Could you check a few things on this model? Use its own coordinates, in mm. Face numbers are marked on the shaded views. A direction names the side the tool comes from. Give positions to 0.01 mm unless a question says otherwise; leave off trailing zeros. Loops run counter-clockwise (first coordinate to the right, second up) from the corner with the lowest first, then second, coordinate; pieces in that order, holes last. Notation, with made-up numbers: (-20, 57) - (-13, 57) arc R21 ccw to (-13, 90) - close; hole circle Ø3 at (47.25, 34.5). An arc over 180 degrees is marked (long way). One line per item, written item: value. Start each with the question number.
Q1. I want a section at D-D (y = 30.5). Please give me the cut outline in (x, z), then the cut area to 3 significant figures.
Q2. I want a section at A-A (x = -22). Please give me the cut outline in (y, z), then the cut area to 3 significant figures.
Q3. If I drill on line 1 (Y direction, x = -31.25, z = 0.7); line 2 (Y direction, x = -39, z = 1.05); line 3 (Z direction, x = -53.5, y = 52.5), over which ranges is the centre line in solid material (lowest first)? Write a range as from..to.
Q4. I want a section at C-C (x = -46.75). Please give me the cut outline in (y, z).
Q5. I'm going to push flat-ended pins straight in: P1, Ø1.2, axis at x = -7, z = 0.5, coming from the +Y side; P2, Ø0.8, axis at y = 53.5, z = 0.5, coming from the +X side; P3, Ø1.6, axis at y = 53, z = 0.5, coming from the -X side. Where does each tip first touch, or does it pass through?
Q6. I want a section at B-B (z = 9). Please give me the cut outline in (x, y).
Q7. For the marked faces 1 and 2, which set-ups out of +Z, -Z, +X, -X, +Y, -Y let a thin tool reach every point of the face, with its end or its side?
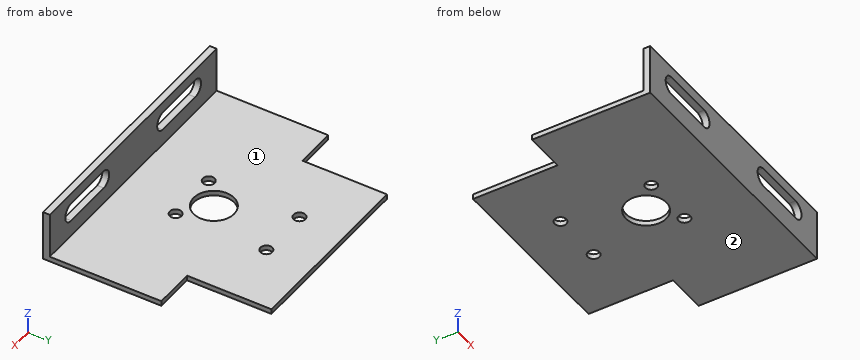
```python
from build123d import *

# Parameters (mm, degrees)
SKETCH_1_R          = 6
SKETCH_1_R_2        = 1.75
EXTRUDE_1_DEPTH     = 1.5
SKETCH_2_W          = 78
SKETCH_2_H          = 2
EXTRUDE_2_DEPTH     = 15
CUT_EXTRUDE_1_DEPTH = 15


with BuildPart() as part:
    # 草图1 → 凸台-拉伸1 (new body)
    with BuildSketch(Plane.XY):
        Polygon((-78, 0), (0, 0), (0, 2), (0, 2.7366), (0, 35), (-12, 35), (-12, 60), (-66, 60), (-66, 35), (-78, 35), (-78, 2.7366), (-78, 2), align=None)
        with Locations((-39, 25.87)):
            Circle(SKETCH_1_R, mode=Mode.SUBTRACT)
        with Locations((-31.25, 19.445882155)):
            Circle(SKETCH_1_R_2, mode=Mode.SUBTRACT)
        with Locations((-46.75, 19.445882155)):
            Circle(SKETCH_1_R_2, mode=Mode.SUBTRACT)
        with Locations((-46.75, 46.292669673)):
            Circle(SKETCH_1_R_2, mode=Mode.SUBTRACT)
        with Locations((-31.25, 46.292669673)):
            Circle(SKETCH_1_R_2, mode=Mode.SUBTRACT)
    extrude(amount=EXTRUDE_1_DEPTH)

    # 草图2 → 凸台-拉伸2 (add)
    with BuildSketch(Plane(origin=(0, 0, 0), x_dir=(-1, 0, 0), z_dir=(0, 0, -1))):
        with Locations((39, 1)):
            Rectangle(SKETCH_2_W, SKETCH_2_H)
    extrude(amount=-EXTRUDE_2_DEPTH)

    # 草图3 → 切除-拉伸1 (cut)
    with BuildSketch(Plane.XZ):
        with BuildLine():
            Line((-68, 11.75), (-52.668833305, 11.75))
            ThreePointArc((-52.668833305, 11.75), (-50.230131523, 9), (-52.668833305, 6.25))
            Line((-52.668833305, 6.25), (-68, 6.25))
            ThreePointArc((-68, 6.25), (-70.75, 9), (-68, 11.75))
        make_face()
        with BuildLine():
            Line((-10, 6.25), (-25.331166695, 6.25))
            ThreePointArc((-25.331166695, 6.25), (-27.769868477, 9), (-25.331166695, 11.75))
            Line((-25.331166695, 11.75), (-10, 11.75))
            ThreePointArc((-10, 11.75), (-7.25, 9), (-10, 6.25))
        make_face()
    extrude(amount=-CUT_EXTRUDE_1_DEPTH, mode=Mode.SUBTRACT)


solid = part.part
```
Worked answers:
1. outline: (-78, 0) - (-42.82, 0) - (-42.82, 1.5) - (-78, 1.5) - close; (-35.18, 0) - (0, 0) - (0, 1.5) - (-35.18, 1.5) - close
1. area: 106 mm²
2. outline: (0, 0) - (60, 0) - (60, 1.5) - (2, 1.5) - (2, 6.25) - (0, 6.25) - close; (0, 11.75) - (2, 11.75) - (2, 15) - (0, 15) - close
2. area: 106 mm²
3. line 1: y = 0..17.7, 21.2..44.54, 48.04..60
3. line 2: y = 0..19.87, 31.87..60
3. line 3: z = 0..1.5
4. outline: (0, 0) - (17.7, 0) - (17.7, 1.5) - (2, 1.5) - (2, 15) - (0, 15) - close; (21.2, 0) - (44.54, 0) - (44.54, 1.5) - (21.2, 1.5) - close; (48.04, 0) - (60, 0) - (60, 1.5) - (48.04, 1.5) - close
5. P1: stops at y = 35
5. P2: stops at x = -12
5. P3: stops at x = -66
6. outline: (-78, 0) - (-70.75, 0) - (-70.75, 2) - (-78, 2) - close; (-50.23, 0) - (-27.77, 0) - (-27.77, 2) - (-50.23, 2) - close; (-7.25, 0) - (0, 0) - (0, 2) - (-7.25, 2) - close
7. face 1: +Z, +X, -X, +Y
7. face 2: -Z, +X, -X, +Y, -Y
